Can you work these out from the model? Positions are in its coordinate system, mm. Face numbers are marked on the shaded views. A direction names the side the tool comes from. Coordinates: 2 decimals unless noted, no trailing zeros. Loops run counter-clockwise (first coordinate to the right, second up) from the corner with the lowest first, then second, coordinate; pieces in that order, holes last.
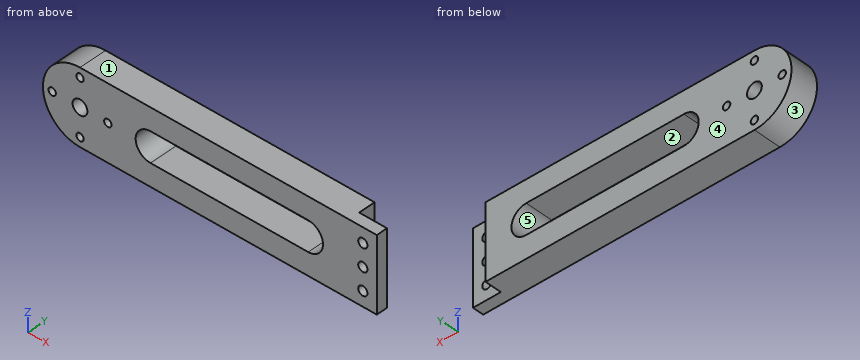
```python
from build123d import *

# Parameters (mm, degrees)
SKETCH_1_R            = 2
SKETCH_1_R_2          = 4
EXTRUDE_1_DEPTH       = 15
CUT_EXTRUDE_1_REACH   = 167.605
SKETCH_2_W            = 15
SKETCH_2_H            = 9
HOLE_WIZARD_5_0_5_1_D = 5
CUT_EXTRUDE_2_REACH   = 163.941


with BuildPart() as part:
    # 草图1 → 凸台-拉伸1 (new body)
    with BuildSketch(Plane(origin=(0, 0, 0), x_dir=(1, 0, 0), z_dir=(0, 1, 0))):
        with BuildLine():
            Line((0, 20), (160, 20))
            Line((160, 20), (160, -20))
            Line((160, -20), (0, -20))
            ThreePointArc((0, -20), (-20, 0), (0, 20))
        make_face()
        with Locations(Location((0, 15, 0), (0, 0, 270))):
            Circle(SKETCH_1_R, mode=Mode.SUBTRACT)
        with Locations(Location((15, 0, 0), (0, 0, 270))):
            Circle(SKETCH_1_R, mode=Mode.SUBTRACT)
        with Locations(Location((0, -15, 0), (0, 0, 270))):
            Circle(SKETCH_1_R, mode=Mode.SUBTRACT)
        with Locations(Location((-15, 0, 0), (0, 0, 270))):
            Circle(SKETCH_1_R, mode=Mode.SUBTRACT)
        with Locations(Location((0, 0, 0), (0, 0, 270))):
            Circle(SKETCH_1_R_2, mode=Mode.SUBTRACT)
    extrude(amount=EXTRUDE_1_DEPTH)

    # 草图2 → 切除-拉伸1 (cut, up to next)
    with BuildSketch(Plane.XY.offset(20), mode=Mode.PRIVATE) as cut_extrude_1_sk1:
        with Locations((152.5, 10.5)):
            Rectangle(SKETCH_2_W, SKETCH_2_H)
    cut_extrude_1_tool1 = extrude(cut_extrude_1_sk1.sketch, amount=-CUT_EXTRUDE_1_REACH, mode=Mode.PRIVATE) & part.part
    add(cut_extrude_1_tool1.solids().sort_by_distance((152.5, 10.5, 20))[0], mode=Mode.SUBTRACT)

    # Ø5.0 (5) 直径孔1 (through all)
    with Locations(Plane(origin=(0, 0, 0), x_dir=(-1, 0, 0), z_dir=(0, -1, 0))):
        with Locations((-152.5, -12), (-152.5, 0), (-152.5, 12)):
            Hole(HOLE_WIZARD_5_0_5_1_D / 2)

    # 草图6 → 切除-拉伸2 (cut, up to next)
    with BuildSketch(Plane(origin=(0, 0, 0), x_dir=(1, 0, 0), z_dir=(0, 1, 0)), mode=Mode.PRIVATE) as cut_extrude_2_sk1:
        with BuildLine():
            Line((38, -8), (123, -8))
            ThreePointArc((123, -8), (131, 0), (123, 8))
            Line((123, 8), (38, 8))
            ThreePointArc((38, 8), (30, 0), (38, -8))
        make_face()
    cut_extrude_2_tool1 = extrude(cut_extrude_2_sk1.sketch, amount=CUT_EXTRUDE_2_REACH, mode=Mode.PRIVATE) & part.part
    add(cut_extrude_2_tool1.solids().sort_by_distance((80.5, 0, 0))[0], mode=Mode.SUBTRACT)


solid = part.part
```
Item 1: We'd pull the mould along X, two halves only. Please class the marked faces 3, 4 and 5: +X half, -X half, draft (parallel to the pull), parting line (faces both ways), or undercut.
Results are:
face 3: -X half
face 4: draft
face 5: undercut
Item 2: Suppose I cut it at B-B, the plane x = 15. Please give me the cut outline in (y, z).
Results are:
outline: (0, -20) - (15, -20) - (15, -2) - (0, -2) - close; (0, 2) - (15, 2) - (15, 20) - (0, 20) - close
Item 3: I'm going to push flat-ended pins straight in: P1, Ø1.5, axis at y = 2.5, z = 9.5, coming from the -X side; P2, Ø7, axis at y = 10, z = 5.5, coming from the +X side; P3, Ø16.5, axis at x = 155.5, z = -5.5, coming from the +Y side. Where does each tip first touch, or does it pass through?
Results are:
P1: stops at x = -17.98
P2: stops at x = 145
P3: stops at y = 6
Item 4: Suppose I cut it at C-C, the plane y = 11.5. Please give me the cut outline in (x, z).
Results are:
outline: (0, -20) - (145, -20) - (145, 20) - (0, 20) arc R20 ccw to start; hole circle Ø4 at (-15, 0); hole circle Ø8 at (0, 0); hole circle Ø4 at (0, -15); hole circle Ø4 at (0, 15); hole circle Ø4 at (15, 0); hole (38, -8) - (123, -8) arc R8 ccw to (123, 8) - (38, 8) arc R8 ccw to start
Item 5: On a 3-axis mill with a long thin cutter (end or side, diameter ignored), from which of +Z, -Z, +X, -X, +Y, -Y can I reach the whole of each face in a straight line? I mean the marked faces 1 and 2. Say none if no direction works.
Results are:
face 1: +Z, +X, -X, +Y, -Y
face 2: +Y, -Y
Item 6: Suppose I cut it at D-D, the plane y = 4.5. Count the separate pieces of the cut face and the enclosed holes in it, plus the area to 3 significant figures.
Results are:
separate pieces: 1
enclosed holes: 9
area: 5,310 mm2
Item 7: I need wall thicknesses on line 1 along X through (y, z) = (6.5, 0); line 2 along Z through (x, y) = (93.5, 1.5); line 3 along X through (y, z) = (4.25, -1). Which ranges of each line are inside material? Lowest first, please.
Results are:
line 1: x = -20 to -17, -13 to -4, 4 to 13, 17 to 30, 131 to 145
line 2: z = -20 to -8, 8 to 20
line 3: x = -19.97 to -16.73, -13.27 to -3.87, 3.87 to 13.27, 16.73 to 30.06, 130.94 to 150.21, 154.79 to 160
Item 8: Suppose I cut it at A-A, the plane z = 0. Please give me the cut outline in (x, y).
Results are:
outline: (-20, 0) - (-17, 0) - (-17, 15) - (-20, 15) - close; (-13, 0) - (-4, 0) - (-4, 15) - (-13, 15) - close; (4, 0) - (13, 0) - (13, 15) - (4, 15) - close; (17, 0) - (30, 0) - (30, 15) - (17, 15) - close; (131, 0) - (150, 0) - (150, 6) - (145, 6) - (145, 15) - (131, 15) - close; (155, 0) - (160, 0) - (160, 6) - (155, 6) - close
